```python
from build123d import *

# Parameters (mm, degrees)
CHAMFER_SIZE = 0.25
SKETCH016_W  = 3.3
SKETCH016_H  = 0.6
POCKET_DEPTH = 10


with BuildPart() as part:
    # Sketch → Revolution (revolve)
    with BuildSketch(Plane.XZ):
        Polygon((-1.35, 1.6), (-1.35, 13), (-3.15, 13), (-3.15, 14.5), (0, 14.5), (0, 0), (-1.3, 0), (-1.65, 1.6), align=None)
    revolve(axis=Axis((0, 0, 0), (0, 0, 1)))

    # Chamfer
    chamfer_edges = [part.edges().sort_by_distance(p)[0] for p in [
        (3.15, 0, 14.5),
    ]]
    chamfer(chamfer_edges, length=CHAMFER_SIZE)

    # Sketch016 (on Face8 of Chamfer) → Pocket (cut)
    with BuildSketch(Plane(origin=(0, 0, 0), x_dir=(1, 0, 0), z_dir=(0, 0, -1))):
        Rectangle(SKETCH016_W, SKETCH016_H)
    extrude(amount=-POCKET_DEPTH, mode=Mode.SUBTRACT)


with BuildPart() as part_1:
    # Body placement: moved
    add(part.part.moved(Location((-22.7, 0.7, -1.6))))


solid = part_1.part
```
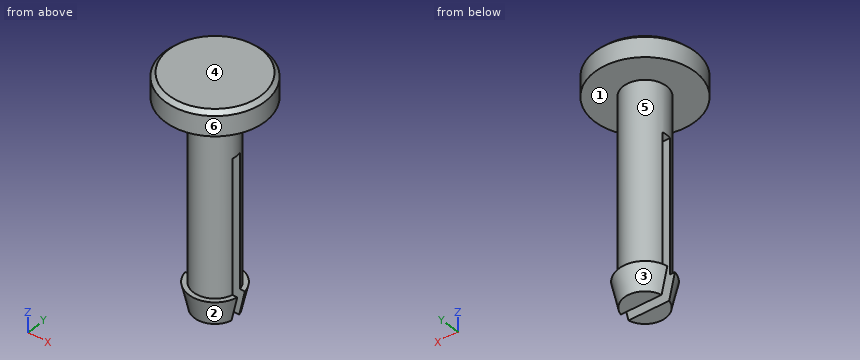
Geometry: final body of the model. Coordinates: model frame, mm. Face numbers are marked on the shaded views. A direction names the side the tool comes from. Give positions to 0.01 mm unless a question says otherwise; leave off trailing zeros. Loops run counter-clockwise (first coordinate to the right, second up) from the corner with the lowest first, then second, coordinate; pieces in that order, holes last. Notation, with made-up numbers: (-20.5, 69) - (-2.5, 69) arc R19 ccw to (-2.5, 85) - close; hole circle Ø10 at (60.25, 65). An arc over 180 degrees is marked (long way). Answer as CSV lines item,"result". Start each with the question number.
(1) Section query D-D (z = 9.5). Output: boundary loops of the cut face in (x, y), and give its area (3 significant figures).
(2) Reachability of the marked faces 1 and 2 from +Z, -Z, +X, -X, +Y, -Y: full face, straight path, thin tool, end or side. Return the list, or none.
(3) Section query C-C (z = 3.5). Output: boundary loops of the cut face in (x, y).
(4) Pin query (flat end, axial travel): P1, Ø2.5, axis at x = -23.5, z = 3, coming from the +Y side; P2, Ø3.5, axis at x = -23, z = 4, coming from the -Y side. Return the tip coordinate at first contact, or that it passes through.
(5) Mould query, pull axis Z, two halves, no side actions, for the marked faces 3, 4, 5 and 6. Classes: +Z half, -Z half, draft (parallel to the pull), parting line (faces both ways), or undercut.
(6) Section query A-A (x = -22.7). Output: boundary loops of the cut face in (y, z).
(7) Section query B-B (y = 0.7). Output: boundary loops of the cut face in (x, z), and give its area (3 significant figures).
(8) Ray query, line 1 along Z through (x, y) = (-20.75, 2.25); line 2 along Z through (x, y) = (-22.5, 0.5); line 3 along Y through (x, z) = (-22, -0.75). Return the intervals inside material, ascending. Write a range as [from, to].
Worked answers:
1,outline,"circle Ø2.7 at (-22.7, 0.7)"
1,area,"5.73 mm^2"
2,face 1,"none"
2,face 2,"-Z, -Y"
3,outline,"(-24.02, 0.4) arc R1.35 ccw to (-21.38, 0.4) - close; (-24.02, 1) - (-21.38, 1) arc R1.35 ccw to start"
4,P1,"stops at y = 2.05"
4,P2,"stops at y = -0.65"
5,face 3,"-Z half"
5,face 4,"+Z half"
5,face 5,"undercut"
5,face 6,"draft"
6,outline,"(-2.45, 11.4) - (-0.65, 11.4) - (-0.65, 0) - (-0.95, 0) - (-0.6, -1.6) - (0.4, -1.6) - (0.4, 8.4) - (1, 8.4) - (1, -1.6) - (2, -1.6) - (2.35, 0) - (2.05, 0) - (2.05, 11.4) - (3.85, 11.4) - (3.85, 12.65) - (3.6, 12.9) - (-2.2, 12.9) - (-2.45, 12.65) - close"
7,outline,"(-25.85, 11.4) - (-24.05, 11.4) - (-24.05, 8.4) - (-21.35, 8.4) - (-21.35, 11.4) - (-19.55, 11.4) - (-19.55, 12.65) - (-19.8, 12.9) - (-25.6, 12.9) - (-25.85, 12.65) - close"
7,area,"17.5 mm^2"
8,line 1,"z = [11.4, 12.9]"
8,line 2,"z = [8.4, 12.9]"
8,line 3,"y = [-0.61, 0.4], [1, 2.01]"
